The listing builds one solid part. Answer for the finished solid, in the listing's coordinates (mm). Give positions to 0.01 mm unless a question says otherwise; leave off trailing zeros. Order: outer loops, then holes, each group sorted by start corner. A loop starts at its lowest first (then second) coordinate and runs counter-clockwise, first axis right, second up.
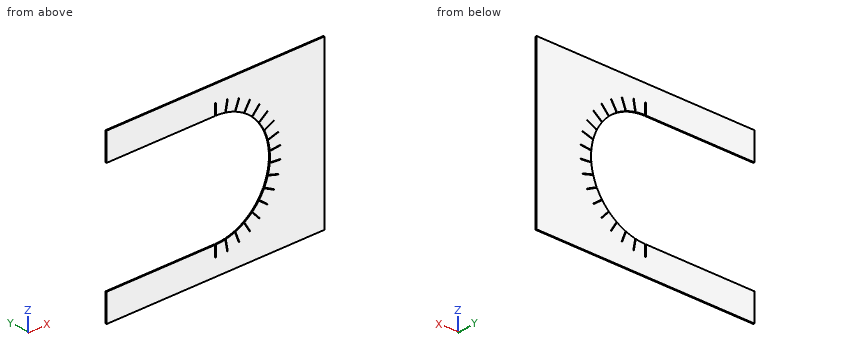
```python
from build123d import *

# Parameters (mm, degrees)
AUFSATZ_LINEAR_AUSTRAGEN1_DEPTH      = 1
SKIZZE2_W                            = 0.5
SKIZZE2_H                            = 15
SCHNITT_LINEAR_AUSTRAGEN_D_NN4_DEPTH = 2
KREISMUSTER12_COUNT                  = 18
KREISMUSTER12_ANGLE                  = 180


with BuildPart() as part:
    # Skizze1 → Aufsatz-Linear austragen1 (new body)
    with BuildSketch(Plane(origin=(0, 0, 0), x_dir=(1, 0, 0), z_dir=(0, 1, 0))):
        with BuildLine():
            Line((0, 50), (-100, 50))
            Line((-100, 50), (-100, 75))
            Line((-100, 75), (100, 75))
            Line((100, 75), (100, -75))
            Line((100, -75), (-100, -75))
            Line((-100, -75), (-100, -50))
            Line((-100, -50), (0, -50))
            ThreePointArc((0, -50), (50, 0), (0, 50))
        make_face()
    extrude(amount=AUFSATZ_LINEAR_AUSTRAGEN1_DEPTH)

    # Skizze2 → Schnitt-Linear-Austragen-Dünn4 (cut)
    with BuildSketch(Plane(origin=(0, 0, 0), x_dir=(1, 0, 0), z_dir=(0, 1, 0))):
        with Locations((0, 52.5)):
            Rectangle(SKIZZE2_W, SKIZZE2_H)
    schnitt_linear_austragen_d_nn4 = extrude(amount=SCHNITT_LINEAR_AUSTRAGEN_D_NN4_DEPTH, mode=Mode.SUBTRACT)

    # Kreismuster12: Schnitt-Linear-Austragen-Dünn4 ×18 about axis
    kreismuster12_axis = Axis((0, 0, 0), (0, -1, 0))
    for i in range(1, KREISMUSTER12_COUNT):
        add(schnitt_linear_austragen_d_nn4.rotate(kreismuster12_axis, i * KREISMUSTER12_ANGLE / (KREISMUSTER12_COUNT - 1)), mode=Mode.SUBTRACT)


solid = part.part
```
1) Given P1, Ø12, axis at x = -27.5, z = 50, coming from the -Y side, flat-ended and moving along its own axis, determine where the tip first touches the part or whether it passes through.
Geometry says:
P1: stops at y = 0
2) Straight lines are drawn through the part: probe 1 along Z at (x, y) = (-77, 0.7); probe 2 along X at (y, z) = (0.55, 58); probe 3 along Z at (x, y) = (40.5, 0.85). For each, find the intervals that lie inside material, in ascending order.
Geometry says:
probe 1: z = -75 to -50, 50 to 75
probe 2: x = -100 to -0.25, 0.25 to 10.59, 11.1 to 100
probe 3: z = -75 to -44.27, -44.06 to -30.9, -30.27 to -29.32, 29.32 to 30.27, 30.9 to 44.06, 44.27 to 75
3) Find section A-A (x = -11). Write down the section's boundary in (y, z).
Geometry says:
outline: (0, -75) - (1, -75) - (1, -50) - (0, -50) - close; (0, 50) - (1, 50) - (1, 75) - (0, 75) - close
